```python
from build123d import *

# Parameters (mm, degrees)
ESBO_O1_R                = 5
ESBO_O1_W                = 12
ESBO_O1_H                = 6
RESSALTO_EXTRUS_O1_DEPTH = 6
RESSALTO_EXTRUS_O2_START = -6
ESBO_O2_R                = 5
ESBO_O2_R_2              = 3
RESSALTO_EXTRUS_O2_DEPTH = 6


with BuildPart() as part:
    # Esboço1 → Ressalto-extrusão1 (new body)
    # profile 1 of 3: a face of its own
    with BuildSketch(Plane.XY):
        with BuildLine():
            ThreePointArc((25.669132457, 72.596513714), (35, 79), (44.330867543, 72.596513714))
            Line((44.330867543, 72.596513714), (70, 6))
            Line((70, 6), (58, 6))
            Line((58, 6), (35, 59))
            Line((35, 59), (12, 6))
            Line((12, 6), (0, 6))
            Line((0, 6), (25.669132457, 72.596513714))
        make_face()
        with Locations((35, 69)):
            Circle(ESBO_O1_R, mode=Mode.SUBTRACT)
    # profile 2 of 3: a face of its own
    with BuildSketch(Plane.XY):
        with Locations((6, 3)):
            Rectangle(ESBO_O1_W, ESBO_O1_H)
    # profile 3 of 3: a face of its own
    with BuildSketch(Plane.XY):
        with Locations((64, 3)):
            Rectangle(ESBO_O1_W, ESBO_O1_H)
    extrude(amount=RESSALTO_EXTRUS_O1_DEPTH)

    # Esboço2 → Ressalto-extrusão2 (add)
    with BuildSketch(Plane.XY.offset(6).offset(RESSALTO_EXTRUS_O2_START)):
        with Locations((35, 69)):
            Circle(ESBO_O2_R)
        with Locations((35, 69)):
            Circle(ESBO_O2_R_2, mode=Mode.SUBTRACT)
    extrude(amount=RESSALTO_EXTRUS_O2_DEPTH)


solid = part.part
```
Here's how the part is built. I have some questions about the finished solid (model axes, mm). A direction names the side the tool comes from. Coordinates: 2 decimals unless noted, no trailing zeros. Write each loop counter-clockwise with the first axis right and the second up, starting at its lowest first coordinate (ties: lowest second). Pieces come first, ordered by that corner, then holes. Notation, with made-up numbers: (25, 23) -> (35, 23) arc R30 cw to (35, 46) -> close; hole circle Ø3 at (39.25, 74). An arc over 180 degrees is marked (long way). Use a Markdown table: item, result. Add a question column.
(1) If we section it at D-D, the plane y = 56: Write out the boundary of the cut face in (x, z).
(2) Please list where these lines run through material, in increasing order: line 1 (Y direction, x = 37.5, z = 3.2); line 2 (X direction, y = 44, z = 4); line 3 (X direction, y = 52, z = 4.4).
(3) For faces 1 (the flat face through (46.66, 32.13, 2.96)), 2 (the flat face through (6, 0, 3)), which set-ups out of +Z, -Z, +X, -X, +Y, -Y let a thin tool reach every point of the face, with its end or its side?
(4) If we section it at A-A, the plane z = 2.25: Write out the boundary of the cut face in (x, y).
(5) I'm going to push flat-ended pins straight in: P1, Ø2, axis at y = 12, z = 1, coming from the +X side; P2, Ø3, axis at x = 54, z = 1, coming from the -Y side; P3, Ø1, axis at y = 46, z = 3.5, coming from the -X side (3 decimals). Where does each tip first touch, or does it pass through?
(6) If we section it at C-C, the plane x = 41.5: Write out the boundary of the cut face in (y, z).
(7) We'd pull the mould along Y, two halves only. Please class faces 3 (the flat face through (23.66, 32.87, 2.96)), 4 (the flat face through (56.986, 39.764, 2.958)), 5 (the cylindrical face through (32.6, 67.2, 3)), 6 (the flat face through (12, 3, 3)): +Y half, -Y half, draft (parallel to the pull), parting line (faces both ways), or undercut.
(8) If we section it at B-B, the plane y = 7: Write out the boundary of the cut face in (x, z).
Outcome:
| question | item | result |
|---|---|---|
| 1 | outline | (19.27, 0) -> (33.7, 0) -> (33.7, 6) -> (19.27, 6) -> close; (36.3, 0) -> (50.73, 0) -> (50.73, 6) -> (36.3, 6) -> close |
| 2 | line 1 | y = 53.24 to 67.34, 70.66 to 78.68 |
| 2 | line 2 | x = 14.65 to 28.49, 41.51 to 55.35 |
| 2 | line 3 | x = 17.73 to 31.96, 38.04 to 52.27 |
| 3 | face 1 | +Z, -Z, -Y |
| 3 | face 2 | +Z, -Z, +X, -X, -Y |
| 4 | outline | (0, 0) -> (12, 0) -> (12, 6) -> (35, 59) -> (58, 6) -> (58, 0) -> (70, 0) -> (70, 6) -> (44.33, 72.6) arc R10 ccw to (25.67, 72.6) -> (0, 6) -> close; hole circle Ø6 at (35, 69) |
| 5 | P1 | stops at x = 68.07 |
| 5 | P2 | stops at y = 11.76 |
| 5 | P3 | stops at x = 15.225 |
| 6 | outline | (44.02, 0) -> (76.6, 0) -> (76.6, 6) -> (44.02, 6) -> close |
| 7 | face 3 | -Y half |
| 7 | face 4 | +Y half |
| 7 | face 5 | undercut |
| 7 | face 6 | draft |
| 8 | outline | (0.39, 0) -> (12.43, 0) -> (12.43, 6) -> (0.39, 6) -> close; (57.57, 0) -> (69.61, 0) -> (69.61, 6) -> (57.57, 6) -> close |
